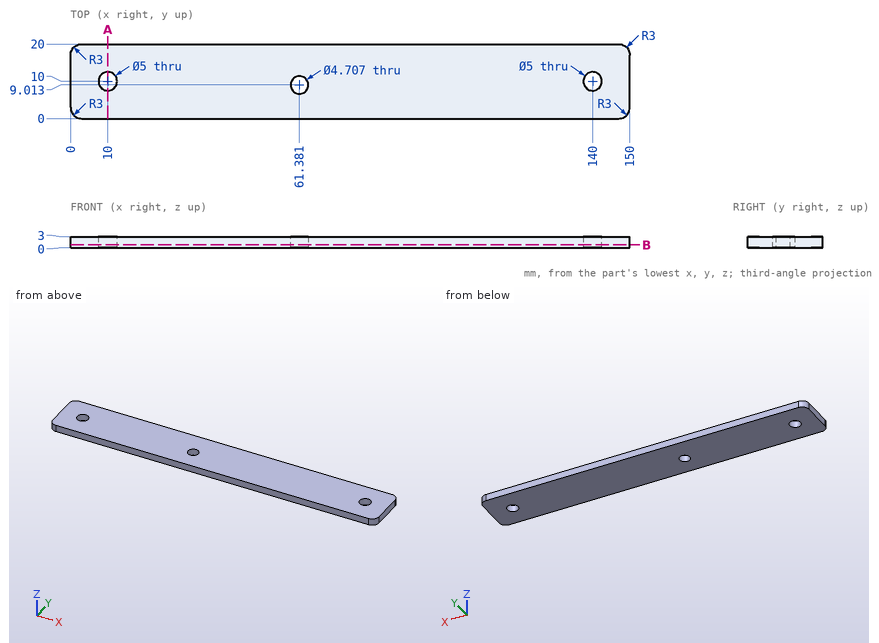
Could you check a few things on this drawing? It's one solid part, dimensions in mm from its lowest x, y, z. Round coordinates to 2 decimals unless told otherwise and drop trailing zeros. Loops run counter-clockwise (first coordinate to the right, second up) from the corner with the lowest first, then second, coordinate; pieces in that order, holes last. Notation, with made-up numbers: (6.5, 51.25) -> (64.5, 51.25) arc R28 cw to (64.5, 70.25) -> close; hole circle Ø7 at (0, -21.5). An arc over 180 degrees is marked (long way). One line per item, written item: value. Start each with the question number.
1. If we section it at A-A, the plane x = 10: Write out the boundary of the cut face in (y, z).
2. If I drill on probe 1 along Y at (x, z) = (10, 0.6); probe 2 along Y at (x, z) = (63, 1.65) (1 decimal); probe 3 along X at (y, z) = (1, 1.05) (1 decimal), over which ranges is the centre line in solid material (lowest first)?
3. If we section it at B-B, the plane z = 0.8: Write out the boundary of the cut face in (x, y) (1 decimal).
Calculated:
1. outline: (0, 0) -> (7.5, 0) -> (7.5, 3) -> (0, 3) -> close; (12.5, 0) -> (20, 0) -> (20, 3) -> (12.5, 3) -> close
2. probe 1: y = 0 to 7.5, 12.5 to 20
2. probe 2: y = 0 to 7.3, 10.7 to 20
2. probe 3: x = 0.8 to 149.2
3. outline: (0, 3) arc R3 ccw to (3, 0) -> (147, 0) arc R3 ccw to (150, 3) -> (150, 17) arc R3 ccw to (147, 20) -> (3, 20) arc R3 ccw to (0, 17) -> close; hole circle Ø5 at (10, 10); hole circle Ø4.7 at (61.4, 9); hole circle Ø5 at (140, 10)
